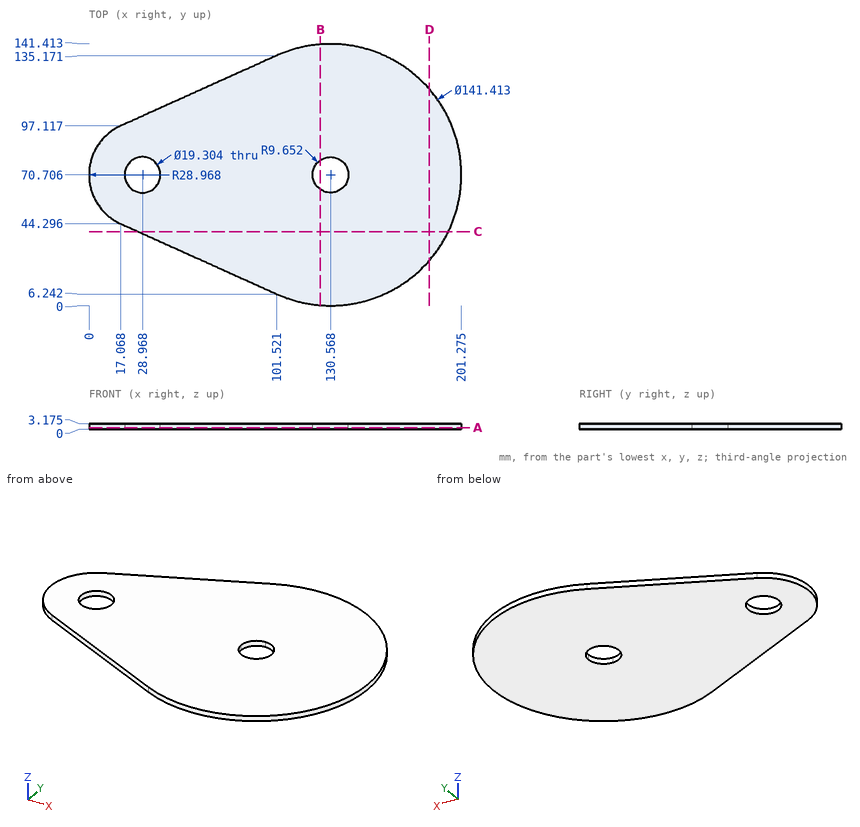
Input: dimensioned drawing with shaded views. Units: mm. Origin: part minimum x, y, z. Round coordinates to 2 decimals unless told otherwise and drop trailing zeros. Order: outer loops, then holes, each group sorted by start corner. A loop starts at its lowest first (then second) coordinate and runs counter-clockwise, first axis right, second up. Notation, with made-up numbers: (60.5, 8) - (104.5, 8) arc R13 ccw to (104.5, 24) - close; hole circle Ø9 at (-4, 24.5). An arc over 180 degrees is marked (long way). Answer as a JSON object with one key per item and string values. Group by question number.
(1) Material intervals for probe 1 along Y at (x, z) = (30, 0.9) (1 decimal); probe 2 along Y at (x, z) = (87, 1.85) (1 decimal); probe 3 along Y at (x, z) = (44, 3), sorted ascending. Write a range as from..to.
(2) Pin query (flat end, axial travel): P1, Ø1, axis at x = 160, z = 1.5, coming from the +Y side; P2, Ø4, axis at x = 54, y = 117.5, coming from the -Z side. Return the tip coordinate at first contact, or that it passes through.
(3) Cut plane D-D (x = 184). Return loops of the section in (y, z) (1 decimal), then the cut area to 3 significant figures.
(4) Cut plane C-C (y = 40). Return loops of the section in (x, z) (1 decimal).
(5) Cut plane B-B (x = 125). Return loops of the section in (y, z) (1 decimal).
(6) Cut plane A-A (z = 1.05). Return loops of the section in (x, y) (1 decimal).
Here are the results:
{
 "1": {"probe 1": "y = 38.5..61.1, 80.3..102.9", "probe 2": "y = 12.8..128.6", "probe 3": "y = 32.16..109.25"},
 "2": {"P1": "stops at y = 135.22", "P2": "passes through"},
 "3": {"outline": "(24.4, 0) - (117, 0) - (117, 3.2) - (24.4, 3.2) - close", "area": "294 mm^2"},
 "4": {"outline": "(26.6, 0) - (194.3, 0) - (194.3, 3.2) - (26.6, 3.2) - close"},
 "5": {"outline": "(0.2, 0) - (62.8, 0) - (62.8, 3.2) - (0.2, 3.2) - close; (78.6, 0) - (141.2, 0) - (141.2, 3.2) - (78.6, 3.2) - close"},
 "6": {"outline": "(17.1, 44.3) - (101.5, 6.2) arc R70.7 ccw (long way) to (101.5, 135.2) - (17.1, 97.1) arc R29 ccw to start; hole circle Ø19.3 at (29, 70.7); hole circle Ø19.3 at (130.6, 70.7)"}
}
